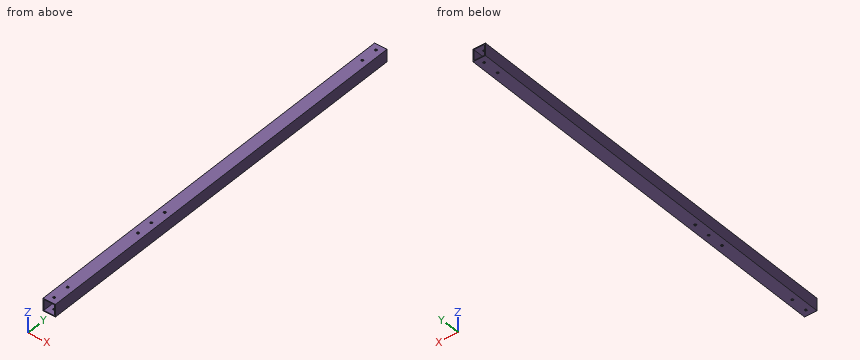
from build123d import *

# Parameters (mm, degrees)
SKETCH_1_W          = 15
SKETCH_1_H          = 15
SKETCH_1_W_2        = 13
SKETCH_1_H_2        = 13
EXTRUDE_1_DEPTH     = 495
SKETCH_2_R          = 1.45
CUT_EXTRUDE_1_DEPTH = 496.284009433


with BuildPart() as part:
    # 草图1 → 拉伸-薄壁1 (new body)
    with BuildSketch(Plane(origin=(0, 0, 0), x_dir=(1, 0, 0), z_dir=(0, 1, 0))):
        Rectangle(SKETCH_1_W, SKETCH_1_H)
        Rectangle(SKETCH_1_W_2, SKETCH_1_H_2, mode=Mode.SUBTRACT)
    extrude(amount=EXTRUDE_1_DEPTH)

    # 草图2 → 切除-拉伸1 (cut, through all)
    with BuildSketch(Plane.XY.offset(7.5)):
        with Locations((0, 487.5)):
            Circle(SKETCH_2_R)
        with Locations((0, 467.5)):
            Circle(SKETCH_2_R)
        with Locations((0, 27.5)):
            Circle(SKETCH_2_R)
        with Locations((0, 7.5)):
            Circle(SKETCH_2_R)
        with Locations((0, 152.5)):
            Circle(SKETCH_2_R)
        with Locations((0, 172.5)):
            Circle(SKETCH_2_R)
        with Locations((0, 132.5)):
            Circle(SKETCH_2_R)
    extrude(amount=-CUT_EXTRUDE_1_DEPTH, mode=Mode.SUBTRACT)


solid = part.part
Source: CAD feature listing. Evaluate the final solid. Frame: model axes, mm. Give positions to 0.01 mm unless a question says otherwise; leave off trailing zeros. Write each loop counter-clockwise with the first axis right and the second up, starting at its lowest first coordinate (ties: lowest second). Pieces come first, ordered by that corner, then holes. Notation, with made-up numbers: M -30,47 L 2,47 A15 cw 2,70 Z; hole C 66.25,-28.5 d11. An arc over 180 degrees is marked long. Return JSON: item names as keys, results as strings. Group by question number.
1) Cut plane B-B, the plane x = 4. Output: boundary loops of the cut face in (y, z).
2) Pin query (flat end, axial travel): P1, Ø2.5, axis at x = 0, y = 467.5, coming from the +Z side. Return the tip coordinate at first contact, or that it passes through.
3) Material intervals for line 1 along Z through (x, y) = (-5.5, 140.5); line 2 along X through (y, z) = (172.5, 7.1), sorted ascending. Write a range as [from, to].
4) Cut plane A-A, the plane z = -2. Output: boundary loops of the cut face in (x, y), plus the area to 3 significant figures.
5) Cut plane C-C, the plane y = 373.5. Output: boundary loops of the cut face in (x, z).
Recorded:
{
 "1": {"outline": "M 0,-7.5 L 495,-7.5 L 495,-6.5 L 0,-6.5 Z; M 0,6.5 L 495,6.5 L 495,7.5 L 0,7.5 Z"},
 "2": {"P1": "passes through"},
 "3": {"line 1": "z = [-7.5, -6.5], [6.5, 7.5]", "line 2": "x = [-7.5, -1.45], [1.45, 7.5]"},
 "4": {"outline": "M -7.5,0 L -6.5,0 L -6.5,495 L -7.5,495 Z; M 6.5,0 L 7.5,0 L 7.5,495 L 6.5,495 Z", "area": "990 mm²"},
 "5": {"outline": "M -7.5,-7.5 L 7.5,-7.5 L 7.5,7.5 L -7.5,7.5 Z; hole M -6.5,-6.5 L 6.5,-6.5 L 6.5,6.5 L -6.5,6.5 Z"}
}
